Verification items for the finished model (mm, model axes). Coordinates: 2 decimals unless noted, no trailing zeros. Loops run counter-clockwise (first coordinate to the right, second up) from the corner with the lowest first, then second, coordinate; pieces in that order, holes last. Notation, with made-up numbers: (-16, 13.5) - (31, 13.5) arc R16 ccw to (31, 35.5) - close; hole circle Ø1 at (-38.75, 68.5). An arc over 180 degrees is marked (long way). Answer as CSV lines item,"result". Start each with the question number.
1. Cross-section at B-B (y = 1.2). State how many separate pieces and enclosed holes the cut face has, plus the area to 3 significant figures.
2. Cross-section at A-A (x = 16). Enter the section's corners in (y, z).
3. Material ranges on line 1 (Z direction, x = -22, y = 1.15); line 2 (Z direction, x = 24, y = 1.9); line 3 (Z direction, x = -49, y = 1.2), recorded low to high. Write a range as [from, to].
4. Gauge pin test, flat end, axial feed: P1, Ø0.5, axis at y = 1.5, z = -3.5, coming from the -X side. Record the tip position at first contact, or that the pin passes through.
5. Release check for a two-part mould opening along Z. For faces 1 (the flat face through (14.4, 1.5, -5.6)), 2 (the flat face through (-1, 2, -4)), 3 (the cylindrical face through (-74.363, 1.493, -4.324)) record: pulls with the +Z half, pulls with the -Z half, needs draft (parallel to the pull), parting line crosses it, or undercut.
```python
from build123d import *

# Parameters (mm, degrees)
BOSS_EXTRUDE1_DEPTH = 2
SKETCH2_W           = 68.264560608
SKETCH2_H           = 24
CUT_EXTRUDE2_DEPTH  = 1.9
RIB1_REACH          = 78.511
SKETCH4_W           = 200.105791224
SKETCH4_H           = 76.194128196
CUT_EXTRUDE3_DEPTH  = 1


with BuildPart() as part:
    # Sketch1 → Boss-Extrude1 (new body)
    with BuildSketch(Plane(origin=(0, 0, 0), x_dir=(1, 0, 0), z_dir=(0, 1, 0))):
        with BuildLine():
            Line((-60, 15), (60, 15))
            ThreePointArc((60, 15), (75, 0), (60, -15))
            Line((60, -15), (42, -15))
            Line((42, -15), (40, -13))
            Line((40, -13), (40, -8.5))
            ThreePointArc((40, -8.5), (41.464466094, -4.964466094), (45, -3.5))
            Line((45, -3.5), (50, -3.5))
            ThreePointArc((50, -3.5), (53.5, 0), (50, 3.5))
            Line((50, 3.5), (37.479805119, 3.5))
            ThreePointArc((37.479805119, 3.5), (33.944271213, 2.035533906), (32.479805119, -1.5))
            Line((32.479805119, -1.5), (32.479805119, -13))
            Line((32.479805119, -13), (30.479805119, -15))
            Line((30.479805119, -15), (-58, -15))
            Line((-58, -15), (-60, -13))
            Line((-60, -13), (-60, -8.5))
            ThreePointArc((-60, -8.5), (-58.535533906, -4.964466094), (-55, -3.5))
            Line((-55, -3.5), (-49.284755489, -3.5))
            ThreePointArc((-49.284755489, -3.5), (-45.784755489, 0), (-49.284755489, 3.5))
            Line((-49.284755489, 3.5), (-62.5, 3.5))
            ThreePointArc((-62.5, 3.5), (-66.035533906, 2.035533906), (-67.5, -1.5))
            Line((-67.5, -1.5), (-67.5, -10.990381057))
            Line((-67.5, -10.990381057), (-68.71685086, -12.207231917))
            ThreePointArc((-68.71685086, -12.207231917), (-74.284755489, 4.576653867), (-60, 15))
        make_face()
    extrude(amount=BOSS_EXTRUDE1_DEPTH)

    # Sketch2 → Cut-Extrude2 (cut)
    with BuildSketch(Plane(origin=(0, 2, 0), x_dir=(1, 0, 0), z_dir=(0, 1, 0))):
        with Locations((-6.652475185, 0)):
            Rectangle(SKETCH2_W, SKETCH2_H)
    extrude(amount=-CUT_EXTRUDE2_DEPTH, mode=Mode.SUBTRACT)

    # Sketch3 walls → Rib1 (add, up to next)
    with BuildSketch(Plane(origin=(0, 2, 0), x_dir=(1, 0, 0), z_dir=(0, 1, 0)), mode=Mode.PRIVATE) as rib1_sk1:
        Polygon((72.690772086, -74.962221531), (10.481384328, 12.862796479), (-6.650895976, -11.137203521), (-23.650895976, 12.862796479), (-86.225903046, -74.796297525), (-85.411999959, -75.377298184), (-23.654054394, 11.137203521), (-6.654054394, -12.862796479), (10.47822591, 11.137203521), (71.874747605, -75.540238871), align=None)
    rib1_tool1 = extrude(rib1_sk1.sketch, amount=-RIB1_REACH, mode=Mode.PRIVATE) - part.part
    # Sketch3 walls → Rib1 (add, up to next)
    with BuildSketch(Plane(origin=(0, 2, 0), x_dir=(1, 0, 0), z_dir=(0, 1, 0)), mode=Mode.PRIVATE) as rib1_sk2:
        Polygon((-86.225903046, 74.796297525), (-23.650895976, -12.862796479), (-6.650895976, 11.137203521), (10.481384328, -12.862796479), (72.690772086, 74.962221531), (71.874747605, 75.540238871), (10.47822591, -11.137203521), (-6.654054394, 12.862796479), (-23.654054394, -11.137203521), (-85.411999959, 75.377298184), align=None)
    rib1_tool2 = extrude(rib1_sk2.sketch, amount=-RIB1_REACH, mode=Mode.PRIVATE) - part.part
    add(rib1_tool1.solids().sort_by_distance((-15.152475185, 2, 0))[0])
    add(rib1_tool2.solids().sort_by_distance((1.913664967, 2, 0))[0])

    # Sketch4 → Cut-Extrude3 (cut)
    with BuildSketch(Plane.XZ):
        with Locations((12.775985132, -7.388521522)):
            Rectangle(SKETCH4_W, SKETCH4_H)
    extrude(amount=-CUT_EXTRUDE3_DEPTH, mode=Mode.SUBTRACT)


solid = part.part
```
Values follow:
1,separate pieces,"1"
1,enclosed holes,"13"
1,area,"2,430 mm²"
2,outline,"(1, -15) - (2, -15) - (2, -12) - (1, -12) - close; (1, -5.07) - (2, -5.07) - (2, -3.34) - (1, -3.34) - close; (1, 3.34) - (2, 3.34) - (2, 5.07) - (1, 5.07) - close; (1, 12) - (2, 12) - (2, 15) - (1, 15) - close"
3,line 1,"z = [-15, -12], [-10.53, -8.8], [8.8, 10.53], [12, 15]"
3,line 2,"z = [-15, -12], [-7.95, -6.22], [6.22, 7.95], [12, 15]"
3,line 3,"z = [-15, -3.49], [3.49, 15]"
4,P1,"stops at x = -74.64"
5,face 1,"undercut"
5,face 2,"needs draft"
5,face 3,"parting line crosses it"
